from build123d import *

# Parameters (mm, degrees)
F0_R     = 2.5
F1_DEPTH = 10
F3_DEPTH = 10
F4_DEPTH = 10
F5_W     = 0.5
F5_H     = 10
F6_DEPTH = 1.5


with BuildPart() as f1:
    # F0 (on Front) → F1 (new body)
    with BuildSketch(Plane.XZ):
        with Locations((-22.092283, 13.107383)):
            Circle(F0_R)
    extrude(amount=F1_DEPTH)

    # F2 (on face) → F3 (cut)
    with BuildSketch(Plane.XZ.offset(10)):
        with BuildLine():
            Line((-20.092283, 11.607383), (-24.092283, 11.607383))
            ThreePointArc((-24.092283, 11.607383), (-22.092283, 10.607383), (-20.092283, 11.607383))
        make_face()
    extrude(amount=-F3_DEPTH, mode=Mode.SUBTRACT)

    # F1_face (on face) → F4 (join)
    with BuildSketch(Plane(origin=(-22.092283, -10, 13.107383), x_dir=(1, 0, 0), z_dir=(0, -1, 0))):
        with BuildLine():
            Line((-2, -1.5), (2, -1.5))
            ThreePointArc((2, -1.5), (0, 2.5), (-2, -1.5))
        make_face()
    extrude(amount=F4_DEPTH)

    # F5 (on face) → F6 (join)
    with BuildSketch(Plane(origin=(0, 0, 11.607383), x_dir=(1, 0, 0), z_dir=(0, 0, -1))):
        with Locations((-24.342283, 15)):
            Rectangle(F5_W, F5_H)
        with Locations((-19.842283, 15)):
            Rectangle(F5_W, F5_H)
    extrude(amount=-F6_DEPTH)


solid = f1.part
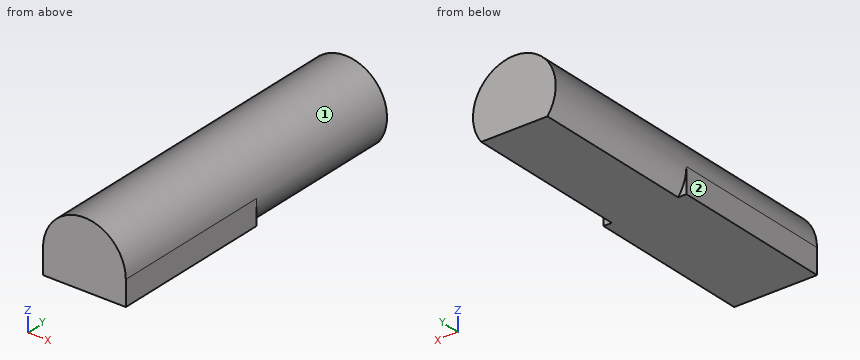
For this review, take the finished solid that the model builds, in its own axes (mm). Face numbers are marked on the shaded views. A direction names the side the tool comes from. Coordinates: 2 decimals unless noted, no trailing zeros. Order: outer loops, then holes, each group sorted by start corner. A loop starts at its lowest first (then second) coordinate and runs counter-clockwise, first axis right, second up. Notation, with made-up numbers: (47.25, -5) -> (67.25, -5) arc R16 cw to (67.25, 0) -> close; hole circle Ø3 at (-13, 28.25). An arc over 180 degrees is marked (long way). Return JSON: item names as keys, results as strings.
1. For pin 1 Ø1.5 at (y, z) = (-17.5, 15) entering from -X; pin 2 Ø1 at (x, y) = (-23, -6) entering from +Z, all flat-tipped, find the tip position at first contact; note any pin that passes through.
Answer block:
{"pin 1": "x = -24.32", "pin 2": "z = 15.57"}
2. Machinability: for the marked faces 1 and 2, which of the approach directions +Z, -Z, +X, -X, +Y, -Y give a long, thin tool a straight path to every point of the face, cutting with its end or side? Answer none if there is none.
Answer block:
{"face 1": "+Y", "face 2": "+Z, -Z, -X, +Y, -Y"}
3. For line 1 (X direction, y = -3.5, z = 13); line 2 (Z direction, x = -24, y = -5.25); line 3 (Z direction, x = -22.6, y = -15.25), list the stretches that pass through material, from the lowest coordinate up. Write a range as from..to.
Answer block:
{"line 1": "-24.59..-19.59", "line 2": "11.61..14.72", "line 3": "11.61..15.56"}
4. We need section A-A on z = 12.2. Write out the cut boundary in (x, y), and give its area (3 significant figures).
Answer block:
{"outline": "(-24.59, -20) -> (-19.59, -20) -> (-19.59, -10) -> (-19.76, -10) -> (-19.76, 0) -> (-24.42, 0) -> (-24.42, -10) -> (-24.59, -10) -> close", "area": "96.6 mm²"}
5. We need section B-B on y = -12.25. Write out the cut boundary in (x, z), and give its area (3 significant figures).
Answer block:
{"outline": "(-24.59, 11.61) -> (-19.59, 11.61) -> (-19.59, 13.11) arc R2.5 ccw to (-24.59, 13.11) -> close", "area": "17.3 mm²"}
6. We need section D-D on y = -9.5. Write out the cut boundary in (x, z), and give its area (3 significant figures).
Answer block:
{"outline": "(-24.09, 11.61) -> (-20.09, 11.61) arc R2.5 ccw (long way) to start", "area": "16.8 mm²"}
7. We need section C-C on x = -23.8. Write out the cut boundary in (y, z), and give its area (3 significant figures).
Answer block:
{"outline": "(-20, 11.61) -> (0, 11.61) -> (0, 14.93) -> (-20, 14.93) -> close", "area": "66.5 mm²"}
